Verification items for the finished model (mm, model axes). A direction names the side the tool comes from. Give positions to 0.01 mm unless a question says otherwise; leave off trailing zeros. Order: outer loops, then holes, each group sorted by start corner. A loop starts at its lowest first (then second) coordinate and runs counter-clockwise, first axis right, second up. Notation, with made-up numbers: (72, -12.75) -> (122, -12.75) arc R4 cw to (122, -6.75) -> close; hole circle Ø3 at (45, -4). An arc over 180 degrees is marked (long way). One line per question, with ' | ' between items. Start each with the question number.
Q1. Section check C-C on y = 0. Give the number of separate pieces and of enclosed holes in the cut face, plus the area to 3 significant figures.
Q2. Section check A-A on z = 5. Record the cut outline in (x, y).
Q3. Access from +Z, -Z, +X, -X, +Y, -Y to the whole of each face (thin tool, end or side, straight path). Record for faces 1 (the cylindrical face through (-2.539, -19.334, 1.479)), 2 (the cylindrical face through (6.691, 12.864, 1.479)), 3 (the flat face through (15.921, -6.595, 16.003)).
Q4. Section check D-D on z = 49. Record the cut outline in (x, y), plus the area to 3 significant figures.
Q5. Mould release check, pull along Y, two halves, no side actions. Record for faces 4 (the flat face through (-13, 9, 60)), 5 (the cylindrical face through (11.376, 11.251, 16.003)), 6 (the cylindrical face through (-18.28, -28.67, 1.48)), 7 (the flat face through (-15.953, -6.608, 16.003)): released by +Y, released by -Y, zero draft, split by the parting line, or undercut.
Q6. Section check B-B on z = 18. Record the cut outline in (x, y), plus the area to 3 significant figures.
Q7. Material ranges on probe 1 along Y at (x, z) = (0, 1.8); probe 2 along X at (y, z) = (0, 45.5), recorded low to high. Write a range as [from, to].
Q8. Go/stop test with flat-tipped pins: pin 1 (1.5 mm diameter, centred on x = 3, z = 54, fed in from -Y); pin 2 (8 mm diameter, centred on x = 21.5, y = 12.5, fed in from -Z); pin 3 (4 mm diameter, centred on x = -5, y = 20, fed in from +Z); pin 4 (1.5 mm diameter, centred on x = 23.5, y = 6.5, fed in from +Z). Record where each tip stops, or that it passes through.
from build123d import *

# Parameters (mm, degrees)
F4_R     = 19.5
F4_R_2   = 14.5
F5_DEPTH = 3
F6_R     = 2.5
F8_R     = 10
F9_R     = 5
F10_R    = 5


with BuildPart() as f1:
    # F0 (on Front) → F1 (revolve)
    with BuildSketch(Plane.XZ):
        Polygon((-34, 0), (-30, 0), (-30, 12.6905989232), (-34, 15), align=None)
        Polygon((-34, 15), (-30, 12.6905989232), (-15.5, 29.9710260159), (-19.5, 32.2804270926), align=None)
        Polygon((-19.5, 32.2804270926), (-15.5, 29.9710260159), (-15.5, 60), (-19.5, 60), align=None)
    revolve(axis=Axis((0, 0, 34.7761163735), (0, 0, 1)))

    # F2 (on face) → F3 (join, up to the next surface of F1)
    with BuildSketch(Plane(origin=(0, 0, 0), x_dir=(1, 0, 0), z_dir=(0, 0, -1))):
        with BuildLine():
            ThreePointArc((-6.1229349178, -14.7820725202), (-11.313708499, -11.313708499), (-14.7820725202, -6.1229349178))
            Line((-14.7820725202, -6.1229349178), (-17.0917713515, -7.0796434988))
            ThreePointArc((-17.0917713515, -7.0796434988), (-13.081475452, -13.081475452), (-7.0796434988, -17.0917713515))
            Line((-7.0796434988, -17.0917713515), (-6.1229349178, -14.7820725202))
        make_face()
        with BuildLine():
            ThreePointArc((7.0796434988, -17.0917713515), (13.081475452, -13.081475452), (17.0917713515, -7.0796434988))
            Line((17.0917713515, -7.0796434988), (14.7820725202, -6.1229349178))
            ThreePointArc((14.7820725202, -6.1229349178), (11.313708499, -11.313708499), (6.1229349178, -14.7820725202))
            Line((6.1229349178, -14.7820725202), (7.0796434988, -17.0917713515))
        make_face()
        with BuildLine():
            Line((-17.0917713515, 7.0796434988), (-14.7820725202, 6.1229349178))
            ThreePointArc((-14.7820725202, 6.1229349178), (-11.313708499, 11.313708499), (-6.1229349178, 14.7820725202))
            Line((-6.1229349178, 14.7820725202), (-7.0796434988, 17.0917713515))
            ThreePointArc((-7.0796434988, 17.0917713515), (-13.081475452, 13.081475452), (-17.0917713515, 7.0796434988))
        make_face()
        with BuildLine():
            Line((14.7820725202, 6.1229349178), (17.0917713515, 7.0796434988))
            ThreePointArc((17.0917713515, 7.0796434988), (13.081475452, 13.081475452), (7.0796434988, 17.0917713515))
            Line((7.0796434988, 17.0917713515), (6.1229349178, 14.7820725202))
            ThreePointArc((6.1229349178, 14.7820725202), (11.313708499, 11.313708499), (14.7820725202, 6.1229349178))
        make_face()
    extrude(until=Until.NEXT, dir=(0, 0, 1))

    # F4 (on face) → F5 (join)
    with BuildSketch(Plane(origin=(0, 0, 0), x_dir=(1, 0, 0), z_dir=(0, 0, -1))):
        Circle(F4_R)
        Circle(F4_R_2, mode=Mode.SUBTRACT)
    extrude(amount=-F5_DEPTH)

    # F6 (on Front) → F7 (revolve, cut)
    with BuildSketch(Plane.XZ):
        with Locations((35.5, 5)):
            Circle(F6_R)
    revolve(axis=Axis((0, 0, 1.7348565161), (0, 0, 1)), mode=Mode.SUBTRACT)

    # F8
    f8_edges = [f1.edges().sort_by_distance(p)[0] for p in [
        (30, 0, 12.690599),
    ]]
    fillet(f8_edges, radius=F8_R)

    # F9
    f9_edges = [f1.edges().sort_by_distance(p)[0] for p in [
        (34, 0, 15),
    ]]
    fillet(f9_edges, radius=F9_R)

    # F10
    f10_edges = [f1.edges().sort_by_distance(p)[0] for p in [
        (19.5, 0, 32.280427),
    ]]
    fillet(f10_edges, radius=F10_R)


solid = f1.part
Filled in:
1) separate pieces: 4 | enclosed holes: 0 | area: 574 mm²
2) outline: circle Ø66 at (0, 0); (-17.09, -7.08) arc R18.5 ccw to (-7.08, -17.09) -> (-6.12, -14.78) arc R16 cw to (-14.78, -6.12) -> close; (-17.09, 7.08) -> (-14.78, 6.12) arc R16 cw to (-6.12, 14.78) -> (-7.08, 17.09) arc R18.5 ccw to start; (6.12, -14.78) -> (7.08, -17.09) arc R18.5 ccw to (17.09, -7.08) -> (14.78, -6.12) arc R16 cw to start; (6.12, 14.78) arc R16 cw to (14.78, 6.12) -> (17.09, 7.08) arc R18.5 ccw to (7.08, 17.09) -> close; hole circle Ø60 at (0, 0)
3) face 1: -Z | face 2: +Z, -Z | face 3: none
4) outline: circle Ø39 at (0, 0); hole circle Ø31 at (0, 0) | area: 440 mm²
5) face 4: zero draft | face 5: undercut | face 6: split by the parting line | face 7: undercut
6) outline: circle Ø62.97 at (0, 0); (-17.09, -7.08) arc R18.5 ccw to (-7.08, -17.09) -> (-6.12, -14.78) arc R16 cw to (-14.78, -6.12) -> close; (-17.09, 7.08) -> (-14.78, 6.12) arc R16 cw to (-6.12, 14.78) -> (-7.08, 17.09) arc R18.5 ccw to start; (6.12, -14.78) -> (7.08, -17.09) arc R18.5 ccw to (17.09, -7.08) -> (14.78, -6.12) arc R16 cw to start; (6.12, 14.78) arc R16 cw to (14.78, 6.12) -> (17.09, 7.08) arc R18.5 ccw to (7.08, 17.09) -> close; hole circle Ø51.09 at (0, 0) | area: 1,200 mm²
7) probe 1: [-34, -30], [-19.5, -14.5], [14.5, 19.5], [30, 34] | probe 2: [-19.5, -15.5], [15.5, 19.5]
8) pin 1: y = -19.37 | pin 2: z = 13.67 | pin 3: z = 60 | pin 4: z = 27.36
